Work out the finished part from the listing and answer in its coordinate system (mm). Give positions to 0.01 mm unless a question says otherwise; leave off trailing zeros. Write each loop counter-clockwise with the first axis right and the second up, starting at its lowest first coordinate (ties: lowest second). Pieces come first, ordered by that corner, then holes. Notation, with made-up numbers: (-28, 37) -> (15, 37) arc R14 ccw to (15, 62) -> close; hole circle Ø3 at (64, 39.5). An arc over 180 degrees is marked (long way). Write item = value, one per line. Start each with the question number.
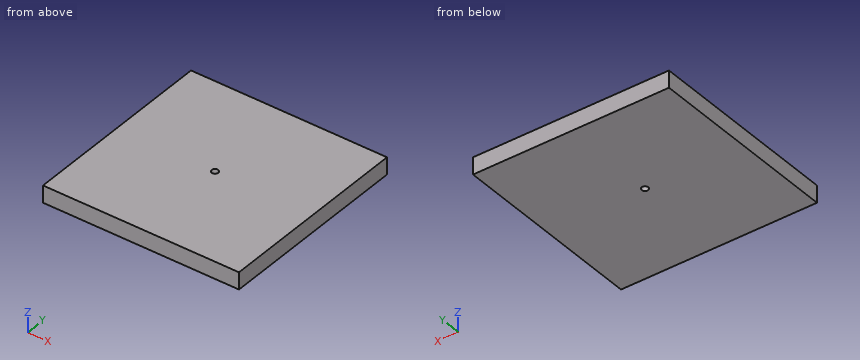
from build123d import *

# Parameters (mm, degrees)
F0_W     = 38.2953807712
F0_H     = 3.3215386793
F1_DEPTH = 38.3032
F4_D     = 1.27


with BuildPart() as f1:
    # F0 (on Front) → F1 (new body)
    with BuildSketch(Plane.XZ):
        Rectangle(F0_W, F0_H)
    extrude(amount=F1_DEPTH)


with BuildPart() as f1_1:
    # F2: moved
    add(f1.part.moved(Location((0, 19.1516, 0))))

    # F4 (through all)
    with Locations(Plane(origin=(0, 0, -1.6607693397), x_dir=(1, 0, 0), z_dir=(0, 0, -1))):
        with Locations((0, 0)):
            Hole(F4_D / 2)


solid = f1_1.part
(1) A cutting plane is placed at A-A, the plane x = 0. Write down the section's boundary in (y, z) (3 decimals), then the cut area to 3 significant figures.
(2) A cutting plane is placed at B-B, the plane y = 0. Write down the section's boundary in (x, z) (3 decimals), then the cut area to 3 significant figures.
(3) Find the intervals of material crossed by line 1 along Y through (x, z) = (0, 0.05) (3 decimals), in increasing order.
Results list:
q1.outline = (-19.152, -1.661) -> (-0.635, -1.661) -> (-0.635, 1.661) -> (-19.152, 1.661) -> close; (0.635, -1.661) -> (19.152, -1.661) -> (19.152, 1.661) -> (0.635, 1.661) -> close
q1.area = 123 mm²
q2.outline = (-19.148, -1.661) -> (-0.635, -1.661) -> (-0.635, 1.661) -> (-19.148, 1.661) -> close; (0.635, -1.661) -> (19.148, -1.661) -> (19.148, 1.661) -> (0.635, 1.661) -> close
q2.area = 123 mm²
q3.line_1 = -19.152 to -0.635, 0.635 to 19.152
